Geometry: final body of the model. Coordinates: model frame, mm. Coordinates: 2 decimals unless noted, no trailing zeros. Loops run counter-clockwise (first coordinate to the right, second up) from the corner with the lowest first, then second, coordinate; pieces in that order, holes last. Notation, with made-up numbers: (-21, -14.75) - (26, -14.75) arc R31 ccw to (26, 19.25) - close; hole circle Ø3 at (12, 71.5). An arc over 180 degrees is marked (long way). Return JSON: item names as keys, results as strings.
from build123d import *

# Parameters (mm, degrees)
SKETCH2_R           = 3
BOSS_EXTRUDE2_DEPTH = 2.5


with BuildPart() as part:
    # Sketch2 → Boss-Extrude2 (new, symmetric)
    # profile 1 of 2: a face of its own
    with BuildSketch(Plane(origin=(0, 0, 0), x_dir=(1, 0, 0), z_dir=(0, 1, 0))):
        Polygon((-2.886751346, -5), (2.886751346, -5), (5.773502692, 0), (2.886751346, 5), (-2.886751346, 5), (-5.773502692, 0), align=None)
        Circle(SKETCH2_R, mode=Mode.SUBTRACT)
    # profile 2 of 2: a face of its own
    with BuildSketch(Plane(origin=(0, 0, 0), x_dir=(1, 0, 0), z_dir=(0, 1, 0))):
        Circle(SKETCH2_R)
    extrude(amount=BOSS_EXTRUDE2_DEPTH, both=True)


solid = part.part
Item 1: Ray query, probe 1 along X at (y, z) = (0.35, 1.75); probe 2 along X at (y, z) = (-0.35, 3); probe 3 along Z at (x, y) = (-3.25, 2.1). Return the intervals inside material, ascending. Write a range as from..to.
Worked out:
{"probe 1": "-4.76..4.76", "probe 2": "-4.04..4.04", "probe 3": "-4.37..4.37"}
Item 2: First-contact query: pin 1 Ø2 at (y, z) = (0, 0.5) entering from +X; pin 2 Ø2 at (y, z) = (1, 1.5) entering from +X; pin 3 Ø1 at (y, z) = (-0.5, 2.5) entering from -X. Flat tips, straight axial feed; report the tip coordinate or a pass-through.
Worked out:
{"pin 1": "x = 5.77", "pin 2": "x = 5.48", "pin 3": "x = -4.62"}
Item 3: Section query A-A, the plane y = 1.55. Return loops of the section in (x, z).
Worked out:
{"outline": "(-5.77, 0) - (-2.89, -5) - (2.89, -5) - (5.77, 0) - (2.89, 5) - (-2.89, 5) - close"}
Item 4: Section query C-C, the plane x = 4.75. Return loops of the section in (y, z), and give its area (3 significant figures).
Worked out:
{"outline": "(-2.5, -1.77) - (2.5, -1.77) - (2.5, 1.77) - (-2.5, 1.77) - close", "area": "17.7 mm^2"}
Item 5: Section query B-B, the plane z = 1.5. Return loops of the section in (x, y).
Worked out:
{"outline": "(-4.91, -2.5) - (4.91, -2.5) - (4.91, 2.5) - (-4.91, 2.5) - close"}
